from build123d import *

# Parameters (mm, degrees)
SKETCH1_R           = 5
BOSS_EXTRUDE1_DEPTH = 15
SKETCH2_R           = 2.5
CUT_EXTRUDE1_DEPTH  = 15
FILLET1_R           = 0.25


with BuildPart() as part:
    # Sketch1 → Boss-Extrude1 (new body)
    with BuildSketch(Plane(origin=(0, 0, 0), x_dir=(1, 0, 0), z_dir=(0, 1, 0))):
        Circle(SKETCH1_R)
    extrude(amount=BOSS_EXTRUDE1_DEPTH)

    # Sketch2 → Cut-Extrude1 (cut)
    with BuildSketch(Plane(origin=(0, 15, 0), x_dir=(1, 0, 0), z_dir=(0, 1, 0))):
        Circle(SKETCH2_R)
    extrude(amount=-CUT_EXTRUDE1_DEPTH, mode=Mode.SUBTRACT)

    # Fillet1
    fillet1_edges = [part.edges().sort_by_distance(p)[0] for p in [
        (-5, 0, 0),
        (-5, 15, 0),
    ]]
    fillet(fillet1_edges, radius=FILLET1_R)


solid = part.part
Work out the finished part from the listing and answer in its coordinate system (mm). Give positions to 0.01 mm unless a question says otherwise; leave off trailing zeros. Order: outer loops, then holes, each group sorted by start corner. A loop starts at its lowest first (then second) coordinate and runs counter-clockwise, first axis right, second up. Notation, with made-up numbers: M 15.25,68.5 L 64.25,68.5 A24 ccw 64.25,84.5 Z; hole C 34,-30.5 d8. An arc over 180 degrees is marked long. Return JSON: item names as keys, results as strings.
Q1. Find the intervals of material crossed by line 1 along X through (y, z) = (9.75, 0); line 2 along X through (y, z) = (6, -0.5), in increasing order. Write a range as [from, to].
Answer below:
{"line 1": "x = [-5, -2.5], [2.5, 5]", "line 2": "x = [-4.97, -2.45], [2.45, 4.97]"}
Q2. Find section B-B, the plane x = 0. Write down the section's boundary in (y, z).
Answer below:
{"outline": "M 0,-4.75 A0.25 ccw 0.25,-5 L 14.75,-5 A0.25 ccw 15,-4.75 L 15,-2.5 L 0,-2.5 Z; M 0,2.5 L 15,2.5 L 15,4.75 A0.25 ccw 14.75,5 L 0.25,5 A0.25 ccw 0,4.75 Z"}
Q3. Find section A-A, the plane z = 0. Write down the section's boundary in (x, y), and give its area (3 significant figures).
Answer below:
{"outline": "M -5,0.25 A0.25 ccw -4.75,0 L -2.5,0 L -2.5,15 L -4.75,15 A0.25 ccw -5,14.75 Z; M 2.5,0 L 4.75,0 A0.25 ccw 5,0.25 L 5,14.75 A0.25 ccw 4.75,15 L 2.5,15 Z", "area": "74.9 mm^2"}
Q4. Each of these flat-tipped pins is pushed along its axis until it touches: pin 1 (5 mm diameter, centred on x = -3.5, y = 9, fed in from +Z); pin 2 (1 mm diameter, centred on x = -3.5, y = 2, fed in from +Z). Where does it stop, or does it pass through?
Answer below:
{"pin 1": "stops at z = 4.9", "pin 2": "stops at z = 4"}
Q5. Find section C-C, the plane y = 13.25. Write down the section's boundary in (x, z).
Answer below:
{"outline": "C 0,0 d10; hole C 0,0 d5"}
Q6. The mould has two halves that part along X. Classify faces 1 (the face through (-1.08, 7.4, 4.88)), 2 (the face through (-0.54, 7.6, 2.44)), 3 (the face through (2, 0, 2)): pulls with the +X half, pulls with the -X half, needs draft (parallel to the pull), parting line crosses it, or undercut.
Answer below:
{"face 1": "parting line crosses it", "face 2": "undercut", "face 3": "needs draft"}
